Geometry: final body of the model. Coordinates: model frame, mm. A direction names the side the tool comes from. Round coordinates to 2 decimals unless told otherwise and drop trailing zeros. Write each loop counter-clockwise with the first axis right and the second up, starting at its lowest first coordinate (ties: lowest second). Pieces come first, ordered by that corner, then holes. Notation, with made-up numbers: M 3,57 L 10,57 A11 cw 10,69 Z; hole C 12.5,40 d2. An arc over 180 degrees is marked long. Use one line per item in the form item = value. Start each with the question number.
from build123d import *

# Parameters (mm, degrees)
SKETCH1_R               = 8.001
BOSS_EXTRUDE1_DEPTH     = 25.4
SKETCH2_R               = 8.001
SKETCH2_R_2             = 6.35
SKETCH2_R_3             = 4.699
CUT_EXTRUDE1_DEPTH      = 12.7
CUT_EXTRUDE4_DEPTH      = 4.1275
CUT_EXTRUDE4_DEPTH_BACK = 12.7
SKETCH5_W               = 21.214200292
SKETCH5_H               = 8.255
CUT_EXTRUDE5_REACH      = 29.806
SKETCH6_R               = 1.5
FILLET2_R               = 1.27
FILLET3_R               = 1.27
CUT_EXTRUDE6_REACH      = 20.919
SKETCH7_R               = 1.25


with BuildPart() as part:
    # Sketch1 → Boss-Extrude1 (new body)
    with BuildSketch(Plane(origin=(0, 0, 0), x_dir=(1, 0, 0), z_dir=(0, 1, 0))):
        with Locations(Location((0, 0, 0), (0, 0, 270))):
            Circle(SKETCH1_R)
    extrude(amount=BOSS_EXTRUDE1_DEPTH)

    # Sketch2 → Cut-Extrude1 (cut)
    # profile 1 of 2: a face of its own
    with BuildSketch(Plane(origin=(0, 0, 0), x_dir=(-1, 0, 0), z_dir=(0, -1, 0))):
        with Locations(Location((0, 0, 0), (0, 0, 90))):
            Circle(SKETCH2_R)
        with Locations(Location((0, 0, 0), (0, 0, 90))):
            Circle(SKETCH2_R_2, mode=Mode.SUBTRACT)
    # profile 2 of 2: a face of its own
    with BuildSketch(Plane(origin=(0, 0, 0), x_dir=(-1, 0, 0), z_dir=(0, -1, 0))):
        with Locations(Location((0, 0, 0), (0, 0, 90))):
            Circle(SKETCH2_R_3)
    extrude(amount=-CUT_EXTRUDE1_DEPTH, mode=Mode.SUBTRACT)

    # Sketch5 → Cut-Extrude4 (cut, two sides: drawn at the far end of the back side and taken through both)
    with BuildSketch(Plane.XY.offset(-CUT_EXTRUDE4_DEPTH_BACK)):
        with Locations((0.442410985, 19.289926646)):
            Rectangle(SKETCH5_W, SKETCH5_H)
    extrude(amount=CUT_EXTRUDE4_DEPTH + CUT_EXTRUDE4_DEPTH_BACK, mode=Mode.SUBTRACT)

    # Sketch6 → Cut-Extrude5 (cut, up to next)
    with BuildSketch(Plane(origin=(0, 25.4, 0), x_dir=(1, 0, 0), z_dir=(0, 1, 0)), mode=Mode.PRIVATE) as cut_extrude5_sk1:
        with Locations(Location((0, 0, 0), (0, 0, 270))):
            Circle(SKETCH6_R)
    cut_extrude5_tool1 = extrude(cut_extrude5_sk1.sketch, amount=-CUT_EXTRUDE5_REACH, mode=Mode.PRIVATE) & part.part
    add(cut_extrude5_tool1.solids().sort_by_distance((0, 25.4, 0))[0], mode=Mode.SUBTRACT)

    # Fillet2
    fillet2_edges = [part.edges().sort_by_distance(p)[0] for p in [
        (0, 23.417426646, 4.1275),
        (0, 15.162426646, 4.1275),
    ]]
    fillet(fillet2_edges, radius=FILLET2_R)

    # Fillet3
    fillet3_edges = [part.edges().sort_by_distance(p)[0] for p in [
        (0, 25.4, -8.001),
    ]]
    fillet(fillet3_edges, radius=FILLET3_R)

    # Sketch7 → Cut-Extrude6 (cut, up to next)
    with BuildSketch(Plane(origin=(0, 15.162426646, 0), x_dir=(1, 0, 0), z_dir=(0, 1, 0)), mode=Mode.PRIVATE) as cut_extrude6_sk1:
        with Locations(Location((0, 0, 0), (0, 0, 270))):
            Circle(SKETCH7_R)
    cut_extrude6_tool1 = extrude(cut_extrude6_sk1.sketch, amount=-CUT_EXTRUDE6_REACH, mode=Mode.PRIVATE) & part.part
    add(cut_extrude6_tool1.solids().sort_by_distance((0, 15.162427, 0))[0], mode=Mode.SUBTRACT)


solid = part.part
1. Section query A-A (z = 0). Return loops of the section in (x, y), then the cut area to 3 significant figures.
2. Set-up query: faces 1 (the face through (0.105, 15.525, 3.746)), 2 (the face through (-1, 12.7, -1)), 3 (the face through (2, 25.4, 0)). Return all of +Z, -Z, +X, -X, +Y, -Y with unobstructed straight access to the full face (end or side cutting, diameter ignored); none if empty.
3. Section query B-B (x = 0). Return loops of the section in (y, z), then the cut area to 3 significant figures.
4. Section query C-C (y = 2.25). Return loops of the section in (x, z), then the cut area to 3 significant figures.
5. Ray query, probe 1 along Y at (x, z) = (-2, -5.5); probe 2 along Y at (x, z) = (-2.5, -0.5); probe 3 along X at (y, z) = (4.25, 0). Return the intervals inside material, ascending.
6. Pull-direction query (X, two-part tool) for faces 4 (the face through (0.45, 24.42, 1.43)), 5 (the face through (-3.86, 6.26, 5.04)), 6 (the face through (0, 23.417, -3)); classes: released by +X, released by -X, zero draft, split by the parting line, or undercut.
7. Contact query for flat-ended pins moving along their axis: pin 1 (4.5 mm diameter, centred on x = 0, z = -2, fed in from -Y); pin 2 (8 mm diameter, centred on y = 8, z = -2, fed in from -X); pin 3 (5 mm diameter, centred on x = -1, z = 3, fed in from -Y); pin 4 (6.5 mm diameter, centred on x = -2, y = 19, fed in from -Z). Output: stop coordinate, or through.
Checks:
q1.outline = M -8,12.7 L -6.35,12.7 L -6.35,0 L -4.7,0 L -4.7,12.7 L -1.25,12.7 L -1.25,15.16 L -8,15.16 Z; M -8,23.42 L -1.5,23.42 L -1.5,25.4 L -6.73,25.4 A1.27 ccw -8,24.13 Z; M 1.25,12.7 L 4.7,12.7 L 4.7,0 L 6.35,0 L 6.35,12.7 L 8,12.7 L 8,15.16 L 1.25,15.16 Z; M 1.5,23.42 L 8,23.42 L 8,24.13 A1.27 ccw 6.73,25.4 L 1.5,25.4 Z
q1.area = 100 mm^2
q2.face_1 = -Z, +X, -X
q2.face_2 = -Y
q2.face_3 = +Z, -Z, +X, -X, +Y
q3.outline = M 0,-6.35 L 12.7,-6.35 L 12.7,-8 L 15.16,-8 L 15.16,-1.25 L 12.7,-1.25 L 12.7,-4.7 L 0,-4.7 Z; M 0,4.7 L 12.7,4.7 L 12.7,1.25 L 15.16,1.25 L 15.16,2.86 A1.27 cw 16.43,4.13 L 22.15,4.13 A1.27 cw 23.42,2.86 L 23.42,1.5 L 25.4,1.5 L 25.4,6.73 A1.27 ccw 24.13,8 L 12.7,8 L 12.7,6.35 L 0,6.35 Z; M 23.42,-8 L 24.13,-8 A1.27 ccw 25.4,-6.73 L 25.4,-1.5 L 23.42,-1.5 Z
q3.area = 133 mm^2
q4.outline = C 0,0 d12.7; hole C 0,0 d9.4
q4.area = 57.3 mm^2
q5.probe_1 = 0 to 15.16, 23.42 to 25.4
q5.probe_2 = 12.7 to 15.16, 23.42 to 25.4
q5.probe_3 = -6.35 to -4.7, 4.7 to 6.35
q6.face_4 = undercut
q6.face_5 = split by the parting line
q6.face_6 = zero draft
q7.pin_1 = 12.7
q7.pin_2 = -6.35
q7.pin_3 = 0
q7.pin_4 = 3.93
